Here's how the part is built. I have some questions about the finished solid (model axes, mm). Give positions to 0.01 mm unless a question says otherwise; leave off trailing zeros. Loops run counter-clockwise (first coordinate to the right, second up) from the corner with the lowest first, then second, coordinate; pieces in that order, holes last. Notation, with made-up numbers: (46.25, -34) - (86.25, -34) arc R18 ccw to (86.25, -28) - close; hole circle Ø2 at (87.5, 43.5). An arc over 180 degrees is marked (long way). Use one line per item in the form item = value.
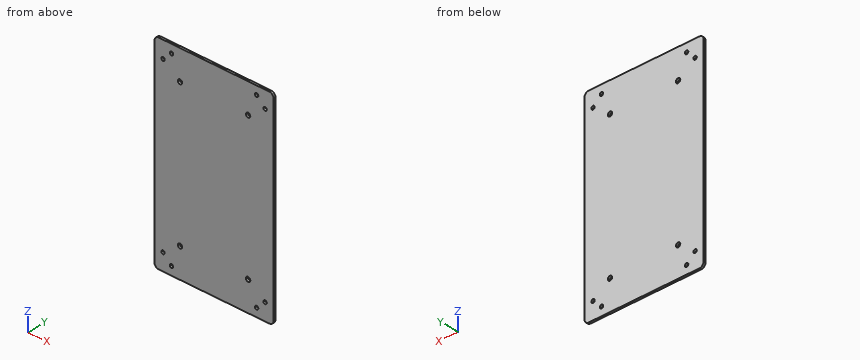
Autodesk Inventor part; units mm, degrees
ref_plane "YZ Plane" through (0, 0, 0) normal (1, 0, 0) x (0, 1, 0)
ref_plane "XZ Plane" through (0, 0, 0) normal (0, 1, 0) x (-1, 0, 0)
ref_plane "XY Plane" through (0, 0, 0) normal (0, 0, 1) x (1, 0, 0)
sketch "Sketch1" plane through (0, 0, 0) normal (0, 1, 0) x (-1, 0, 0)
  line L0 (88.9, -152.4) -> (-88.9, -152.4)
  line L1 (-88.9, -152.4) -> (-88.9, 152.4)
  line L2 (-88.9, 152.4) -> (88.9, 152.4)
  line L3 (88.9, 152.4) -> (88.9, -152.4)
  line L4 (88.9, -152.4) -> (-88.9, 152.4) construction
  line L5 (-88.9, -152.4) -> (88.9, 152.4) construction
  point P0 (0, 0)
  dimension "d0" = 177.8
  dimension "d1" = 304.8
extrude "Plate1" add sketch "Sketch1" along normal blind 3.175
fillet "Corner Round1" radius 6.35 4 edges at (-88.9, 1.5875, 152.4) (88.9, 1.5875, 152.4) (-88.9, 1.5875, -152.4) (88.9, 1.5875, -152.4)
sketch "Sketch2" plane through (0, 3.175, 0) normal (0, 1, 0) x (1, 0, 0)
  circle A0 centre (-76.2, 127) radius 2.5797
  line L0 (-88.9, -146.05) -> (-88.9, 146.05)
  line L1 (-82.55, 152.4) -> (82.55, 152.4)
  circle A1 centre (-63.5, 139.7) radius 2.5797
  line L2 (-88.9, 0) -> (88.9, 0) construction
  line L3 (88.9, 146.05) -> (88.9, -146.05) construction
  line L4 (-82.55, 152.4) -> (82.55, 152.4) construction
  line L5 (0, 152.4) -> (0, -152.4) construction
  line L6 (82.55, -152.4) -> (-82.55, -152.4) construction
  circle A2 centre (76.2, 127) radius 2.5797
  circle A3 centre (63.5, 139.7) radius 2.5797
  circle A4 centre (-76.2, -127) radius 2.5797
  circle A5 centre (-63.5, -139.7) radius 2.5797
  circle A6 centre (63.5, -139.7) radius 2.5797
  circle A7 centre (76.2, -127) radius 2.5797
  circle A8 centre (-50.8, 107.95) radius 3.302
  line L7 (-50.8, 107.95) -> (50.8, 107.95) construction
  circle A9 centre (50.8, 107.95) radius 3.302
  line L8 (50.8, 107.95) -> (50.8, -107.95) construction
  circle A10 centre (50.8, -107.95) radius 3.302
  line L9 (50.8, -107.95) -> (-50.8, -107.95) construction
  circle A11 centre (-50.8, -107.95) radius 3.302
  line L10 (-50.8, 107.95) -> (-50.8, -107.95) construction
  point P0 (0, 0)
  point P1 (0, 107.95)
  point P2 (-50.8, 0)
  dimension "d4" = 5.1594
  dimension "d5" = 12.7
  dimension "d6" = 25.4
  dimension "d7" = 12.7
  dimension "d8" = 25.4
  dimension "d11" = 101.6
  dimension "d12" = 6.604
  dimension "d13" = 215.9
extrude "Cut1" cut sketch "Sketch2" against normal blind 3.175
equation "\"d9\" = Thickness"
equation "\"d2\" = Thickness"
equation "\"BendRadius\" = 1.5 * Thickness"
equation "\"BendReliefWidth\" = Thickness"
equation "\"BendReliefDepth\" = 0.5 * Thickness"
equation "\"CornerReliefSize\" = 4 * Thickness"
equation "\"MinimumRemnant\" = 2 * Thickness"
equation "\"TransitionRadius\" = BendRadius"
equation "\"JacobiRadiusSize\" = BendRadius"
equation "\"GapSize\" = Thickness"
properties part number "PDP_Plate" material "Aluminum 5052 H32"
(1) If we section it at A-A (x = -50.8): List the corners of the cut face in (y, z) for me (3 decimals).
Geometry says:
outline = (0, -152.4) - (3.175, -152.4) - (3.175, -111.252) - (0, -111.252) - close; (0, -104.648) - (3.175, -104.648) - (3.175, 104.648) - (0, 104.648) - close; (0, 111.252) - (3.175, 111.252) - (3.175, 152.4) - (0, 152.4) - close
(2) If we section it at B-B (z = 107.95): List the corners of the cut face in (x, y) for me (3 decimals), plus the area to 3 significant figures.
Geometry says:
outline = (-88.9, 0) - (-54.102, 0) - (-54.102, 3.175) - (-88.9, 3.175) - close; (-47.498, 0) - (47.498, 0) - (47.498, 3.175) - (-47.498, 3.175) - close; (54.102, 0) - (88.9, 0) - (88.9, 3.175) - (54.102, 3.175) - close
area = 523 mm²
(3) If I drill on probe 1 along Z at (x, y) = (-76.2, 2); probe 2 along X at (y, z) = (0.7, 127); probe 3 along Z at (x, y) = (-63.5, 0.7), over which ranges is the centre line in solid material (lowest first)?
Geometry says:
probe_1 = -152.4 to -129.58, -124.42 to 124.42, 129.58 to 152.4
probe_2 = -88.9 to -78.78, -73.62 to 73.62, 78.78 to 88.9
probe_3 = -152.4 to -142.28, -137.12 to 137.12, 142.28 to 152.4
